Input: part model. Units: mm. Frame: model coordinates. A direction names the side the tool comes from. Round coordinates to 2 decimals unless told otherwise and drop trailing zeros. Loops run counter-clockwise (first coordinate to the right, second up) from the corner with the lowest first, then second, coordinate; pieces in that order, holes last. Notation, with made-up numbers: (7.5, -31) -> (59.5, -31) arc R11 ccw to (59.5, -12) -> close; hole circle Ø11 at (-35.5, 13). An arc over 180 degrees is marked (long way). Answer in a Markdown table with one row per item. Add a question column.
Q1. Ray query, L1, parallel to Z at x = 66, y = 21; L2, parallel to Z at x = 66.5, y = 12; L3, parallel to Z at x = 31, y = 23.5. Return the intervals inside material, ascending. Write a range as from..to.
Q2. Pin query (flat end, axial travel): pin 1 (10 mm diameter, centred on x = 53.5, z = -9.5, fed in from +Y); pin 2 (14 mm diameter, centred on x = 58.5, y = 17, fed in from +Z); pin 3 (14 mm diameter, centred on y = 12, z = -14, fed in from -X); pin 4 (1.5 mm diameter, centred on x = 11, y = 9, fed in from +Z). Return the tip coordinate at first contact, or that it passes through.
Q3. Reachability of faces 4 (the face through (30.221, 16, -12)), 5 (the face through (89.08, 15.03, -65.68)), 6 (the face through (15.067, 16.314, -65.011)) from +Z, -Z, +X, -X, +Y, -Y: full face, straight path, thin tool, end or side. Return the list, or none.
Q4. Section C-C, the plane z = -9. Output: boundary loops of the cut face in (x, y), and give its area (3 significant figures).
Q5. Section D-D, the plane x = 78. Output: boundary loops of the cut face in (y, z).
Q6. Section A-A, the plane y = 23. Output: boundary loops of the cut face in (x, z).
Q7. Section B-B, the plane x = 41. Output: boundary loops of the cut face in (y, z), and give its area (3 significant figures).
Q8. Mould query, pull axis Z, two halves, no side actions, for faces 1 (the face through (51, 16, -20.32)), 2 (the face through (44, 30.48, -25)), 3 (the face through (12.88, 15.03, -66.3)). Classes: pulls with the +Z half, pulls with the -Z half, needs draft (parallel to the pull), parting line crosses it, or undercut.
```python
from build123d import *

# Parameters (mm, degrees)
BOSS_EXTRUDE1_DEPTH = 2.54
SKETCH3_W           = 36.089649417
SKETCH3_H           = 17.78
SKETCH3_W_2         = 31.009649417
SKETCH3_H_2         = 12.7
BOSS_EXTRUDE2_DEPTH = 30.48


with BuildPart() as part:
    # Sketch2 → Boss-Extrude1 (new body)
    with BuildSketch(Plane(origin=(0, 0, 0), x_dir=(1, 0, 0), z_dir=(0, 1, 0))):
        Polygon((76.2, 0), (101.6, 43.994090512), (76.2, 87.988181024), (25.4, 87.988181024), (0, 43.994090512), (25.4, 0), align=None)
    extrude(amount=BOSS_EXTRUDE1_DEPTH)

    # Sketch3 → Boss-Extrude2 (add)
    with BuildSketch(Plane(origin=(0, 0, 0), x_dir=(1, 0, 0), z_dir=(0, 1, 0))):
        with Locations((50.805939368, 11.43)):
            Rectangle(SKETCH3_W, SKETCH3_H)
        with Locations((50.805939368, 11.43)):
            Rectangle(SKETCH3_W_2, SKETCH3_H_2, mode=Mode.SUBTRACT)
        Polygon((30.221114659, 22.86), (30.221114659, 0), (25.4, 0), (0, 43.994090512), (25.4, 87.988181024), (76.2, 87.988181024), (101.6, 43.994090512), (76.2, 0), (71.390764076, 0), (71.390764076, 22.86), align=None)
        Polygon((73.930764076, 2.54), (74.733530316, 2.54), (98.667060633, 43.994090512), (74.733530316, 85.448181024), (26.866469684, 85.448181024), (2.932939367, 43.994090512), (26.866469684, 2.54), (27.681114659, 2.54), (27.681114659, 25.4), (73.930764076, 25.4), align=None, mode=Mode.SUBTRACT)
    extrude(amount=BOSS_EXTRUDE2_DEPTH)


solid = part.part
```
Answer block:
| question | item | result |
|---|---|---|
| 1 | L1 | -87.99..-85.45, -25.4..-22.86, -20.32..-17.78, -5.08..-2.54 |
| 1 | L2 | -87.99..-85.45, -25.4..-22.86, -20.32..-2.54 |
| 1 | L3 | -87.99..-85.45, -25.4..-22.86 |
| 2 | pin 1 | y = 30.48 |
| 2 | pin 2 | z = -2.54 |
| 2 | pin 3 | x = 13.28 |
| 2 | pin 4 | z = -23.64 |
| 3 | face 4 | +Z, +Y |
| 3 | face 5 | -Z, +X, +Y, -Y |
| 3 | face 6 | +Y |
| 4 | outline | (20.2, 0) -> (81.4, 0) -> (81.4, 30.48) -> (78.46, 30.48) -> (78.46, 2.54) -> (73.93, 2.54) -> (73.93, 30.48) -> (71.39, 30.48) -> (71.39, 2.54) -> (68.85, 2.54) -> (68.85, 30.48) -> (66.31, 30.48) -> (66.31, 2.54) -> (35.3, 2.54) -> (35.3, 30.48) -> (32.76, 30.48) -> (32.76, 2.54) -> (30.22, 2.54) -> (30.22, 30.48) -> (27.68, 30.48) -> (27.68, 2.54) -> (23.14, 2.54) -> (23.14, 30.48) -> (20.2, 30.48) -> close |
| 4 | area | 603 mm^2 |
| 5 | outline | (0, -84.87) -> (30.48, -84.87) -> (30.48, -79.79) -> (2.54, -79.79) -> (2.54, -8.2) -> (30.48, -8.2) -> (30.48, -3.12) -> (0, -3.12) -> close |
| 6 | outline | (0, -43.99) -> (25.4, -87.99) -> (76.2, -87.99) -> (101.6, -43.99) -> (76.2, 0) -> (71.39, 0) -> (71.39, -22.86) -> (30.22, -22.86) -> (30.22, 0) -> (25.4, 0) -> close; (32.76, -20.32) -> (68.85, -20.32) -> (68.85, -2.54) -> (32.76, -2.54) -> close; hole (2.93, -43.99) -> (26.87, -85.45) -> (74.73, -85.45) -> (98.67, -43.99) -> (74.73, -2.54) -> (73.93, -2.54) -> (73.93, -25.4) -> (27.68, -25.4) -> (27.68, -2.54) -> (26.87, -2.54) -> close; hole (35.3, -17.78) -> (66.31, -17.78) -> (66.31, -5.08) -> (35.3, -5.08) -> close |
| 7 | outline | (0, -87.99) -> (30.48, -87.99) -> (30.48, -85.45) -> (2.54, -85.45) -> (2.54, -25.4) -> (30.48, -25.4) -> (30.48, -22.86) -> (2.54, -22.86) -> (2.54, -20.32) -> (30.48, -20.32) -> (30.48, -17.78) -> (2.54, -17.78) -> (2.54, -5.08) -> (30.48, -5.08) -> (30.48, -2.54) -> (2.54, -2.54) -> (2.54, 0) -> (0, 0) -> close |
| 7 | area | 507 mm^2 |
| 8 | face 1 | undercut |
| 8 | face 2 | needs draft |
| 8 | face 3 | pulls with the -Z half |
